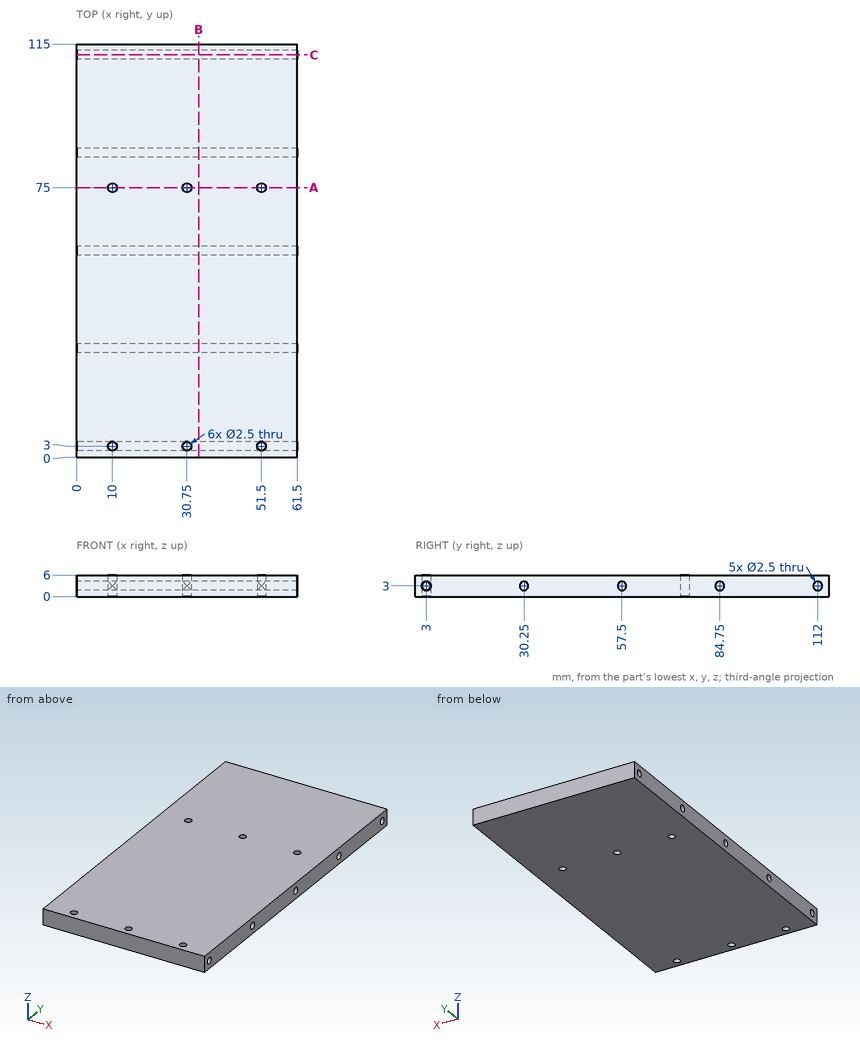
Print and shaded views of the part. All mm, measured from the part's lowest x, y and z. Give positions to 0.01 mm unless a question says otherwise; leave off trailing zeros. Order: outer loops, then holes, each group sorted by start corner. A loop starts at its lowest first (then second) coordinate and runs counter-clockwise, first axis right, second up. Notation, with made-up numbers: M 78,-38 L 131,-38 A21 ccw 131,-8 Z; hole C 32.25,82.25 d9. An arc over 180 degrees is marked long. Use one line per item in the form item = value.
Q1. Slice it at C-C, the plane y = 112. Write the cut outline in (x, z).
Conclusion:
outline = M 0,0 L 61.5,0 L 61.5,1.75 L 0,1.75 Z; M 0,4.25 L 61.5,4.25 L 61.5,6 L 0,6 Z
Q2. Wall check: probe 1 along Y at (x, z) = (30.75, 1); probe 2 along X at (y, z) = (75, 4.4); probe 3 along Y at (x, z) = (54.5, 3). Give the ranges that are in metal, low to high.
Conclusion:
probe_1 = 0 to 1.75, 4.25 to 73.75, 76.25 to 115
probe_2 = 0 to 8.75, 11.25 to 29.5, 32 to 50.25, 52.75 to 61.5
probe_3 = 0 to 1.75, 4.25 to 29, 31.5 to 56.25, 58.75 to 83.5, 86 to 110.75, 113.25 to 115
Q3. Slice it at A-A, the plane y = 75. Write the cut outline in (x, z).
Conclusion:
outline = M 0,0 L 8.75,0 L 8.75,6 L 0,6 Z; M 11.25,0 L 29.5,0 L 29.5,6 L 11.25,6 Z; M 32,0 L 50.25,0 L 50.25,6 L 32,6 Z; M 52.75,0 L 61.5,0 L 61.5,6 L 52.75,6 Z
Q4. Slice it at B-B, the plane x = 34. Write the cut outline in (y, z), and give its area (3 significant figures).
Conclusion:
outline = M 0,0 L 115,0 L 115,6 L 0,6 Z; hole C 3,3 d2.5; hole C 30.25,3 d2.5; hole C 57.5,3 d2.5; hole C 84.75,3 d2.5; hole C 112,3 d2.5
area = 665 mm2
